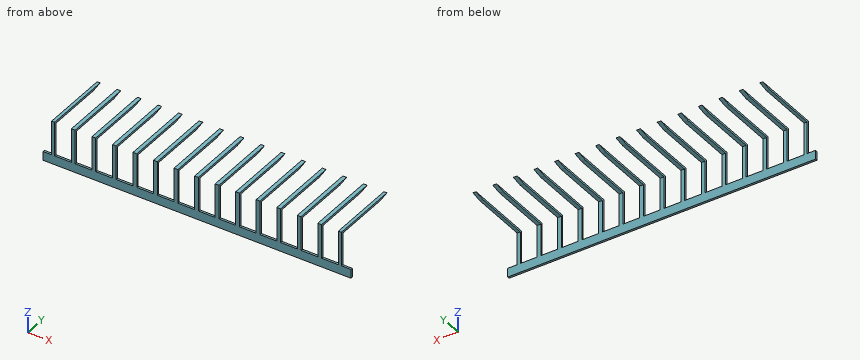
```python
from build123d import *

# Parameters (mm, degrees)
SKETCH_1_W          = 450
SKETCH_1_H          = 60
EXTRUDE_1_DEPTH     = 3
SKETCH_2_W          = 450
SKETCH_2_H          = 100
EXTRUDE_2_DEPTH     = 3
CUT_EXTRUDE_2_DEPTH = 465.865571967
SKETCH_3_W          = 14
SKETCH_3_H          = 50
SKETCH_3_W_2        = 24.5
SKETCH_3_W_3        = 12.5
CUT_EXTRUDE_3_DEPTH = 465.865571967


with BuildPart() as part:
    # 草图1 → 凸台-拉伸1 (new body)
    with BuildSketch(Plane(origin=(0, 0, 0), x_dir=(1, 0, 0), z_dir=(0, 1, 0))):
        with Locations((225, 30)):
            Rectangle(SKETCH_1_W, SKETCH_1_H)
    extrude(amount=EXTRUDE_1_DEPTH)

    # 草图2 → 凸台-拉伸2 (add)
    with BuildSketch(Plane.XY):
        with Locations((225, 50)):
            Rectangle(SKETCH_2_W, SKETCH_2_H)
    extrude(amount=EXTRUDE_2_DEPTH)

    # 草图6 → 切除-拉伸2 (cut, through all)
    with BuildSketch(Plane(origin=(450, 0, 0), x_dir=(0, 0, -1), z_dir=(1, 0, 0))):
        Polygon((-3, 100), (0, 85), (0, 100), align=None)
    extrude(amount=-CUT_EXTRUDE_2_DEPTH, mode=Mode.SUBTRACT)

    # 草图3 → 切除-拉伸3 (cut, through all)
    with BuildSketch(Plane.XZ):
        with Locations((443, -22)):
            Rectangle(SKETCH_3_W, SKETCH_3_H)
        with Locations((419.25, -22)):
            Rectangle(SKETCH_3_W_2, SKETCH_3_H)
        with Locations((389.25, -22)):
            Rectangle(SKETCH_3_W_2, SKETCH_3_H)
        with Locations((359.25, -22)):
            Rectangle(SKETCH_3_W_2, SKETCH_3_H)
        with Locations((329.25, -22)):
            Rectangle(SKETCH_3_W_2, SKETCH_3_H)
        with Locations((299.25, -22)):
            Rectangle(SKETCH_3_W_2, SKETCH_3_H)
        with Locations((269.25, -22)):
            Rectangle(SKETCH_3_W_2, SKETCH_3_H)
        with Locations((239.25, -22)):
            Rectangle(SKETCH_3_W_2, SKETCH_3_H)
        with Locations((209.25, -22)):
            Rectangle(SKETCH_3_W_2, SKETCH_3_H)
        with Locations((179.25, -22)):
            Rectangle(SKETCH_3_W_2, SKETCH_3_H)
        with Locations((149.25, -22)):
            Rectangle(SKETCH_3_W_2, SKETCH_3_H)
        with Locations((119.25, -22)):
            Rectangle(SKETCH_3_W_2, SKETCH_3_H)
        with Locations((89.25, -22)):
            Rectangle(SKETCH_3_W_2, SKETCH_3_H)
        with Locations((59.25, -22)):
            Rectangle(SKETCH_3_W_2, SKETCH_3_H)
        with Locations((29.25, -22)):
            Rectangle(SKETCH_3_W_2, SKETCH_3_H)
        with Locations((6.25, -22)):
            Rectangle(SKETCH_3_W_3, SKETCH_3_H)
    extrude(amount=-CUT_EXTRUDE_3_DEPTH, mode=Mode.SUBTRACT)


solid = part.part
```
For this review, take the finished solid that the model builds, in its own axes (mm). Give positions to 0.01 mm unless a question says otherwise; leave off trailing zeros. Write each loop counter-clockwise with the first axis right and the second up, starting at its lowest first coordinate (ties: lowest second). Pieces come first, ordered by that corner, then holes. Notation, with made-up numbers: M -31,15 L 19,15 A15 ccw 19,35 Z; hole C -20,70.5 d5. An arc over 180 degrees is marked long. Answer as a JSON object with one key per item and string values. Group by question number.
Item 1: For pin 1 Ø3 at (x, y) = (345, 29) entering from -Z; pin 2 Ø4 at (x, y) = (128.5, 27) entering from +Z; pin 3 Ø5 at (x, z) = (196.5, -52.5) entering from +Y; pin 4 Ø0.9 at (x, y) = (215, 1) entering from +Z, all flat-tipped, find the tip position at first contact; note any pin that passes through.
Item 2: Consider section A-A on y = 16. Count the separate pieces of the cut face and the enclosed holes in it, plus the area to 4 significant figures.
Item 3: For probe 1 along Y at (x, z) = (104, -46); probe 2 along Z at (x, y) = (223, 90.5), list the stretches that pass through material, from the lowest coordinate up. Write a range as [from, to].
Item 4: Consider section C-C on x = 388.5. Write out the cut boundary in (y, z), plus the area to 3 significant figures.
Check result:
{
 "1": {"pin 1": "stops at z = 0", "pin 2": "passes through", "pin 3": "stops at y = 3", "pin 4": "stops at z = -47"},
 "2": {"separate pieces": "15", "enclosed holes": "0", "area": "241.5 mm^2"},
 "3": {"probe 1": "y = [0, 3]", "probe 2": "z = [1.1, 3]"},
 "4": {"outline": "M 0,-60 L 3,-60 L 3,-47 L 0,-47 Z", "area": "39.0 mm^2"}
}
